Here's how the part is built. I have some questions about the finished solid (model axes, mm). Round coordinates to 2 decimals unless told otherwise and drop trailing zeros. Loops run counter-clockwise (first coordinate to the right, second up) from the corner with the lowest first, then second, coordinate; pieces in that order, holes last. Notation, with made-up numbers: M -31.5,38.25 L -17.5,38.25 A26 cw -17.5,73.25 Z; hole C -22,70 d5. An arc over 180 degrees is marked long. Use a Markdown table: item, result.
```python
from build123d import *

# Parameters (mm, degrees)
SKETCH_1_W          = 100
SKETCH_1_H          = 80
EXTRUDE_1_DEPTH     = 30
SKETCH_2_R          = 5
CUT_EXTRUDE_1_DEPTH = 5
SKETCH_3_W          = 15
SKETCH_3_H          = 6
CUT_EXTRUDE_2_DEPTH = 5
SKETCH_5_R          = 1.25
CUT_EXTRUDE_3_DEPTH = 51


with BuildPart() as part:
    # 草图1 → 凸台-拉伸1 (new body)
    with BuildSketch(Plane(origin=(0, 0, 0), x_dir=(1, 0, 0), z_dir=(0, 1, 0))):
        Rectangle(SKETCH_1_W, SKETCH_1_H)
    extrude(amount=EXTRUDE_1_DEPTH)

    # 草图2 → 切除-拉伸1 (cut)
    with BuildSketch(Plane(origin=(0, 0, -40), x_dir=(-1, 0, 0), z_dir=(0, 0, -1))):
        with Locations((-41, 9)):
            Circle(SKETCH_2_R)
    extrude(amount=-CUT_EXTRUDE_1_DEPTH, mode=Mode.SUBTRACT)

    # 草图3 → 切除-拉伸2 (cut)
    with BuildSketch(Plane(origin=(0, 0, -40), x_dir=(-1, 0, 0), z_dir=(0, 0, -1))):
        with Locations((-12.5, 18)):
            Rectangle(SKETCH_3_W, SKETCH_3_H)
        with Locations((12.5, 18)):
            Rectangle(SKETCH_3_W, SKETCH_3_H)
        with Locations((-12.5, 6)):
            Rectangle(SKETCH_3_W, SKETCH_3_H)
        with Locations((12.5, 6)):
            Rectangle(SKETCH_3_W, SKETCH_3_H)
    extrude(amount=-CUT_EXTRUDE_2_DEPTH, mode=Mode.SUBTRACT)

    # 草图5 → 切除-拉伸3 (cut)
    with BuildSketch(Plane.XZ):
        with Locations(Location((46, 36, 0), (0, 0, 270))):
            Circle(SKETCH_5_R)
        with Locations(Location((-40, 36, 0), (0, 0, 270))):
            Circle(SKETCH_5_R)
        with Locations(Location((-40, -22, 0), (0, 0, 270))):
            Circle(SKETCH_5_R)
        with Locations(Location((46, -22, 0), (0, 0, 270))):
            Circle(SKETCH_5_R)
    extrude(amount=-CUT_EXTRUDE_3_DEPTH, mode=Mode.SUBTRACT)


solid = part.part
```
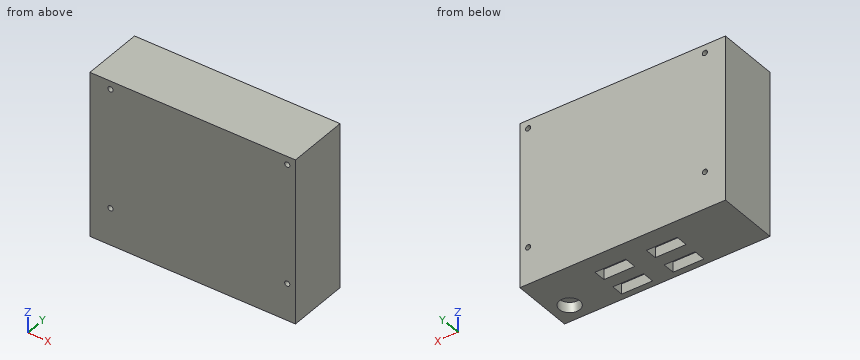
Q1. I need wall thicknesses on line 1 (X direction, y = 9.75, z = 36); line 2 (Z direction, x = 36.5, y = 8.5); line 3 (Y direction, x = 41, z = -38). Which ranges of each line are inside material? Lowest first, please. Write a range as from..to.
Return value:
| item | result |
|---|---|
| line 1 | x = -50..-41.25, -38.75..44.75, 47.25..50 |
| line 2 | z = -35..40 |
| line 3 | y = 0..4, 14..30 |
Q2. Will this pin go through, and if not, where does the flat tip stop? P1, Ø3, axis at x = 41, y = 8, coming from the -Z side.
Return value:
| item | result |
|---|---|
| P1 | stops at z = -35 |
Q3. Imagine slicing it at C-C, the plane x = 41. Please give me the cut outline in (y, z).
Return value:
| item | result |
|---|---|
| outline | M 0,-40 L 4,-40 L 4,-35 L 14,-35 L 14,-40 L 30,-40 L 30,40 L 0,40 Z |
Q4. Imagine slicing it at A-A, the plane z = -22. Please give me the cut outline in (x, y).
Return value:
| item | result |
|---|---|
| outline | M -50,0 L -41.25,0 L -41.25,30 L -50,30 Z; M -38.75,0 L 44.75,0 L 44.75,30 L -38.75,30 Z; M 47.25,0 L 50,0 L 50,30 L 47.25,30 Z |
Q5. Imagine slicing it at B-B, the plane x = -40. Please give me the cut outline in (y, z).
Return value:
| item | result |
|---|---|
| outline | M 0,-40 L 30,-40 L 30,-23.25 L 0,-23.25 Z; M 0,-20.75 L 30,-20.75 L 30,34.75 L 0,34.75 Z; M 0,37.25 L 30,37.25 L 30,40 L 0,40 Z |
Q6. Imagine slicing it at D-D, the plane x = -14. Please give me the cut outline in (y, z).
Return value:
| item | result |
|---|---|
| outline | M 0,-40 L 3,-40 L 3,-35 L 9,-35 L 9,-40 L 15,-40 L 15,-35 L 21,-35 L 21,-40 L 30,-40 L 30,40 L 0,40 Z |
